from build123d import *


with BuildPart() as part:
    # Sketch1 → Revolve1 (revolve)
    with BuildSketch(Plane.XY, mode=Mode.PRIVATE) as revolve1_sk:
        Polygon((-1, 12), (-6, 12), (-6, 16), (-26, 16), (-26, 18), (-6, 18), (-6, 25), (0, 25), (0, 10), (-1, 10), align=None)
    revolve(revolve1_sk.sketch.rotate(Axis((-42.809570876, 0, 0), (1, 0, 0)), 90), axis=Axis((-42.809570876, 0, 0), (1, 0, 0)))


solid = part.part
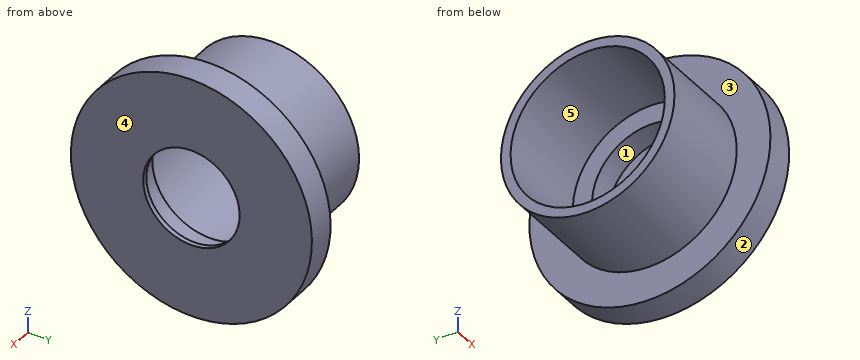
Part model, mm, in its own coordinate system. Face numbers are marked on the shaded views. A direction names the side the tool comes from. Give positions to 0.01 mm unless a question says otherwise; leave off trailing zeros. Order: outer loops, then holes, each group sorted by start corner. A loop starts at its lowest first (then second) coordinate and runs counter-clockwise, first axis right, second up. Notation, with made-up numbers: (-22, 61) - (-3, 61) arc R15 cw to (-3, 76) - close; hole circle Ø4 at (-35.75, 8.25). An arc over 180 degrees is marked (long way). One line per question, with ' | ' between items.
1. Which spindle directions (+Z, -Z, +X, -X, +Y, -Y) get a long thin tool onto all of the face, cutting with end or side? Do the marked faces 4 and 5. Say none if no direction does.
Filled in:
face 4: +Z, -Z, +X, +Y, -Y | face 5: -X
2. Drill centre lines: probe 1 along Y at (x, z) = (-2.1, 0); probe 2 along Y at (x, z) = (-0.5, 0); probe 3 along X at (y, z) = (-10, 4.5). Where is each one in solid material? Low to high.
Filled in:
probe 1: -25 to -12, 12 to 25 | probe 2: -25 to -10, 10 to 25 | probe 3: -1 to 0
3. Band-saw the part on B-B on z = 9. List the corners of the cut face in (x, y).
Filled in:
outline: (-26, -15.59) - (-6, -15.59) - (-6, -23.32) - (0, -23.32) - (0, -4.36) - (-1, -4.36) - (-1, -7.94) - (-6, -7.94) - (-6, -13.23) - (-26, -13.23) - close; (-26, 13.23) - (-6, 13.23) - (-6, 7.94) - (-1, 7.94) - (-1, 4.36) - (0, 4.36) - (0, 23.32) - (-6, 23.32) - (-6, 15.59) - (-26, 15.59) - close
4. Band-saw the part on C-C on x = -17.25. List the corners of the cut face in (y, z), then the cut area to 3 significant figures.
Filled in:
outline: circle Ø36 at (0, 0); hole circle Ø32 at (0, 0) | area: 214 mm²
5. Pull direction Z, two halves, no side cores. Call the marked faces 1, 2 and 3: +Z half, -Z half, draft (parallel to the pull), parting line (faces both ways), or undercut.
Filled in:
face 1: undercut | face 2: parting line | face 3: draft
6. Band-saw the part on D-D on z = -15. List the corners of the cut face in (x, y), then the cut area to 3 significant figures.
Filled in:
outline: (-26, -9.95) - (-6, -9.95) - (-6, -20) - (0, -20) - (0, 20) - (-6, 20) - (-6, 9.95) - (-26, 9.95) - (-26, 5.57) - (-6, 5.57) - (-6, -5.57) - (-26, -5.57) - close | area: 415 mm²
7. Band-saw the part on A-A on y = 0. List the corners of the cut face in (x, z).
Filled in:
outline: (-26, -18) - (-6, -18) - (-6, -25) - (0, -25) - (0, -10) - (-1, -10) - (-1, -12) - (-6, -12) - (-6, -16) - (-26, -16) - close; (-26, 16) - (-6, 16) - (-6, 12) - (-1, 12) - (-1, 10) - (0, 10) - (0, 25) - (-6, 25) - (-6, 18) - (-26, 18) - close
8. Drop flat-ended pins along their axis: P1, Ø9.5, axis at y = -3.5, z = 6, coming from the -X side; P2, Ø1.5, axis at x = -20.5, z = 5, coming from the +Y side; P3, Ø6, axis at x = -7.5, z = 13.5, coming from the +Y side. Give the stop position or say it passes through.
Filled in:
P1: x = -1 | P2: y = 17.49 | P3: y = 22.5
